```python
from build123d import *

# Parameters (mm, degrees)
SKETCH2_R               = 50.8
BOSS_EXTRUDE1_DEPTH     = 4.7625
BOSS_EXTRUDE2_DEPTH     = 30
SKETCH7_W               = 60
SKETCH7_H               = 50
BOSS_EXTRUDE3_DEPTH     = 46.7625
CUT_EXTRUDE2_DEPTH      = 81.8
SKETCH5_W               = 52
SKETCH5_H               = 33.1537
CUT_EXTRUDE1_DEPTH      = 51.8
CUT_EXTRUDE1_DEPTH_BACK = 51.8


with BuildPart() as part:
    # Sketch2 → Boss-Extrude1 (new body)
    with BuildSketch(Plane(origin=(0, 0, 0), x_dir=(-1, 0, 0), z_dir=(0, 1, 0))):
        Circle(SKETCH2_R)
    extrude(amount=BOSS_EXTRUDE1_DEPTH)

    # Sketch4 → Boss-Extrude2 (add, symmetric)
    with BuildSketch(Plane(origin=(0, 0, 0), x_dir=(0, 0, -1), z_dir=(1, 0, 0))):
        Polygon((-25, 4.7625), (25, 4.7625), (16, 46.7625), (-16, 46.7625), align=None)
    extrude(amount=BOSS_EXTRUDE2_DEPTH, both=True)

    # Sketch7 → Boss-Extrude3 (add)
    with BuildSketch(Plane(origin=(0, 0, 0), x_dir=(-1, 0, 0), z_dir=(0, 1, 0))):
        Rectangle(SKETCH7_W, SKETCH7_H)
    extrude(amount=BOSS_EXTRUDE3_DEPTH)

    # Sketch6 → Cut-Extrude2 (cut, through all)
    with BuildSketch(Plane(origin=(30, 0, 0), x_dir=(0, 0, -1), z_dir=(1, 0, 0))):
        with BuildLine():
            Line((5, 40.7625), (5, 46.7625))
            Line((5, 46.7625), (-5, 46.7625))
            Line((-5, 46.7625), (-5, 40.7625))
            ThreePointArc((-5, 40.7625), (0, 35.7625), (5, 40.7625))
        make_face()
    extrude(amount=-CUT_EXTRUDE2_DEPTH, mode=Mode.SUBTRACT)

    # Sketch5 → Cut-Extrude1 (cut, two sides)
    with BuildSketch(Plane.XY) as cut_extrude1_sk:
        with Locations((0, 30.18565)):
            Rectangle(SKETCH5_W, SKETCH5_H)
    extrude(amount=CUT_EXTRUDE1_DEPTH, mode=Mode.SUBTRACT)
    extrude(cut_extrude1_sk.sketch, amount=-CUT_EXTRUDE1_DEPTH_BACK, mode=Mode.SUBTRACT)


solid = part.part
```
Geometry check sheet. Reference: the model listing, model coordinates, mm. A direction names the side the tool comes from. Give positions to 0.01 mm unless a question says otherwise; leave off trailing zeros. Write each loop counter-clockwise with the first axis right and the second up, starting at its lowest first coordinate (ties: lowest second). Pieces come first, ordered by that corner, then holes.
1) Section check A-A, the plane y = 30. Record the boundary of the cut face in (x, z), and give its area (3 significant figures).
2) Section check B-B, the plane x = 0. Record the boundary of the cut face in (y, z).
3) Gauge pin test, flat ends, axial feed: pin 1 (10 mm diameter, centred on x = -23.5, z = 21, fed in from -Y); pin 2 (1.2 mm diameter, centred on x = -28.5, y = 42.5, fed in from -Z); pin 3 (2 mm diameter, centred on x = 28.5, y = 42.5, fed in from +Z); pin 4 (2 mm diameter, centred on x = 12, z = 23, fed in from +Y). Record the tip position at first contact, or that the pin passes through.
4) Access from +Z, -Z, +X, -X, +Y, -Y to the whole of each face (thin tool, end or side, straight path). Record for faces 5 (the flat face through (-26, 30, 0)), 6 (the flat face through (-28, 46.762, 15)), 7 (the flat face through (0, 11, 25)), 8 (the flat face through (30, 26, 0)), 9 (the flat face through (-28, 44, 5)).
5) Release check for a two-part mould opening along X. For faces 1 (the flat face through (-30, 26, 0)), 2 (the cylindrical face through (28.028, 35.764, 0.11)), 3 (the cylindrical face through (11.012, 2.348, -49.592)), 4 (the flat face through (0, 13.609, 0)) record: pulls with the +X half, pulls with the -X half, needs draft (parallel to the pull), parting line crosses it, or undercut.
6) Material ranges on L1, parallel to X at y = 35.5, z = 19; L2, parallel to Y at x = -35, z = 24.5; L3, parallel to Y at x = 21.5, z = -5.5, recorded low to high.
7) Section check D-D, the plane y = 11.5. Record the boundary of the cut face in (x, z), and give its area (3 significant figures).
8) Section check C-C, the plane z = 0. Record the boundary of the cut face in (x, y), and give its area (3 significant figures).
Computed:
1. outline: (-30, -25) - (-26, -25) - (-26, 25) - (-30, 25) - close; (26, -25) - (30, -25) - (30, 25) - (26, 25) - close
1. area: 400 mm2
2. outline: (0, -50.8) - (4.76, -50.8) - (4.76, -25) - (13.61, -25) - (13.61, 25) - (4.76, 25) - (4.76, 50.8) - (0, 50.8) - close
3. pin 1: stops at y = 0
3. pin 2: stops at z = -25
3. pin 3: stops at z = 25
3. pin 4: stops at y = 13.61
4. face 5: +Z, -Z, +Y
4. face 6: +Z, -Z, +X, -X, +Y
4. face 7: +Z, +X, -X, +Y
4. face 8: +Z, -Z, +X, +Y
4. face 9: +X, -X, +Y
5. face 1: pulls with the -X half
5. face 2: needs draft
5. face 3: parting line crosses it
5. face 4: undercut
6. L1: x = -30 to -26, 26 to 30
6. L2: y = 0 to 4.76
6. L3: y = 0 to 13.61
7. outline: (-30, -25) - (30, -25) - (30, 25) - (-30, 25) - close
7. area: 3,000 mm2
8. outline: (-50.8, 0) - (50.8, 0) - (50.8, 4.76) - (30, 4.76) - (30, 35.76) - (26, 35.76) - (26, 13.61) - (-26, 13.61) - (-26, 35.76) - (-30, 35.76) - (-30, 4.76) - (-50.8, 4.76) - close
8. area: 1,190 mm2
